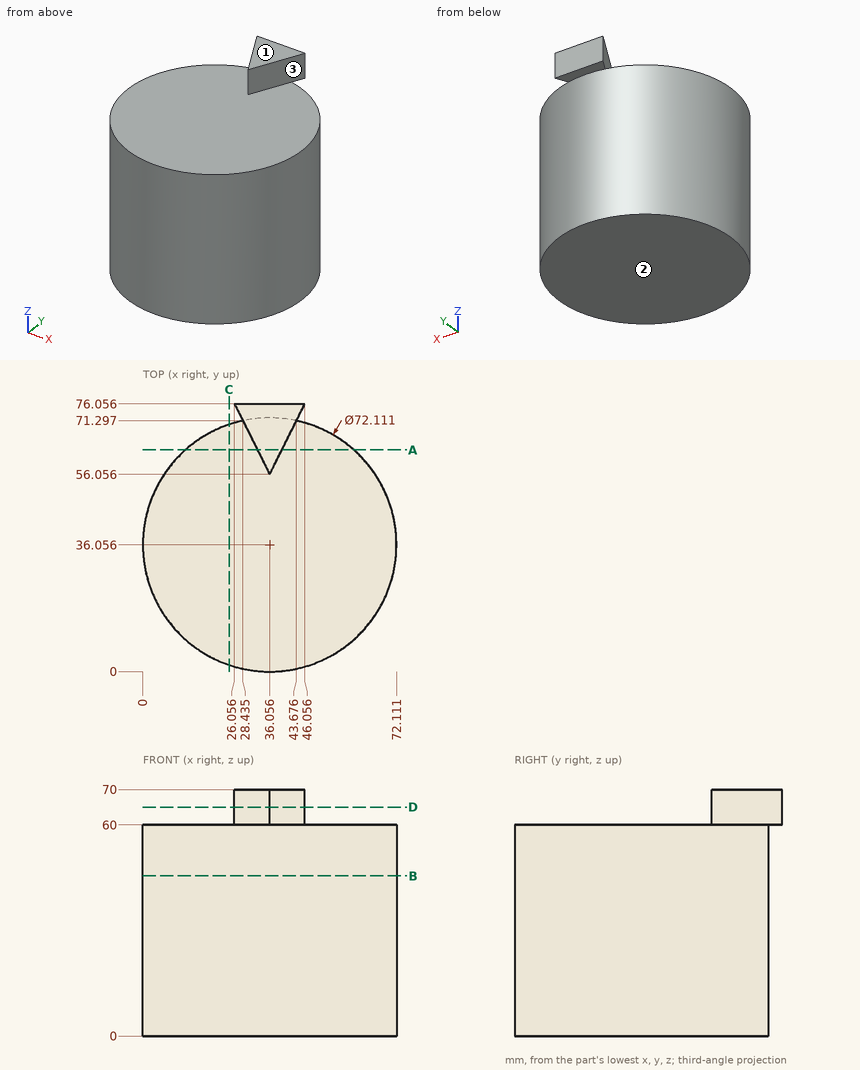
For this review, use the dimensioned drawing (mm, ordinates from the lowest corner) and the shaded views. Coordinates: 2 decimals unless noted, no trailing zeros. Write each loop counter-clockwise with the first axis right and the second up, starting at its lowest first coordinate (ties: lowest second). Pieces come first, ordered by that corner, then holes. Notation, with made-up numbers: (49, 75.5) - (58, 75.5) arc R24 ccw to (58, 98.5) - close; hole circle Ø2 at (-6.75, 84). An arc over 180 degrees is marked (long way). Answer as a JSON object with one key per item and string values. Group by question number.
1. Add section D-D (z = 65). Give the boundary of the cut face in (x, y) (1 decimal), plus the area to 3 significant figures.
2. To check wall thickness, follow probe 1 along Z at (x, y) = (34, 11.5); probe 2 along X at (y, z) = (44, 24) (1 decimal); probe 3 along X at (y, z) = (45, 5.5) (1 decimal). State the ranges of each line that lie inside material, in increasing order.
3. Add section C-C (x = 24.5). Give the boundary of the cut face in (y, z), plus the area to 3 significant figures.
4. Clearance check with flat-ended pins moving along their axes: pin 1 Ø2 at (y, z) = (50.5, 58) entering from -X; pin 2 Ø12 at (y, z) = (13, 30) entering from +X; pin 3 Ø5 at (x, y) = (11.5, 58) entering from +Z. State where each tip first meets the part, or that it passes through.
5. Add section B-B (z = 45.5). Give the boundary of the cut face in (x, y) (1 decimal), plus the area to 3 significant figures.
6. Mouldability with a two-part tool opening along Z and no side actions: class the marked faces 1, 2 and 3 as pulls with the +Z half, pulls with the -Z half, needs draft (parallel to the pull), parting line crosses it, or undercut.
7. Add section A-A (y = 63). Give the boundary of the cut face in (x, z).
Findings:
{
 "1": {"outline": "(26.1, 76.1) - (36.1, 56.1) - (46.1, 76.1) - close", "area": "200 mm²"},
 "2": {"probe 1": "0 to 60", "probe 2": "0.9 to 71.2", "probe 3": "1.1 to 71"},
 "3": {"outline": "(1.9, 0) - (70.21, 0) - (70.21, 60) - (1.9, 60) - close", "area": "4,100 mm²"},
 "4": {"pin 1": "x = 2.6", "pin 2": "x = 67.82", "pin 3": "z = 60"},
 "5": {"outline": "circle Ø72.1 at (36.1, 36.1)", "area": "4,080 mm²"},
 "6": {"face 1": "pulls with the +Z half", "face 2": "pulls with the -Z half", "face 3": "needs draft"},
 "7": {"outline": "(12.1, 0) - (60.01, 0) - (60.01, 60) - (39.53, 60) - (39.53, 70) - (32.58, 70) - (32.58, 60) - (12.1, 60) - close"}
}
